Verification items for the finished model (mm, model axes). Face numbers are marked on the shaded views. A direction names the side the tool comes from. Coordinates: 2 decimals unless noted, no trailing zeros. Write each loop counter-clockwise with the first axis right and the second up, starting at its lowest first coordinate (ties: lowest second). Pieces come first, ordered by that corner, then holes. Notation, with made-up numbers: M 70,-34 L 93,-34 A12 ccw 93,-30 Z; hole C -34.75,66.25 d7. An arc over 180 degrees is marked long. Answer in a Markdown table with one row per item.
from build123d import *

# Parameters (mm, degrees)
F0_W     = 113
F0_H     = 67
F1_DEPTH = 2
F2_W     = 113
F2_H     = 67
F2_W_2   = 101
F2_H_2   = 55
F3_DEPTH = 10
F4_R     = 1.5
F5_DEPTH = 6.25


with BuildPart() as f1:
    # F0 (on Top) → F1 (new body)
    with BuildSketch(Plane.XY):
        Rectangle(F0_W, F0_H)
    extrude(amount=F1_DEPTH)

    # F2 (on face) → F3 (join)
    with BuildSketch(Plane.XY.offset(2)):
        Rectangle(F2_W, F2_H)
        Rectangle(F2_W_2, F2_H_2, mode=Mode.SUBTRACT)
    extrude(amount=F3_DEPTH)

    # F4 (on face) → F5 (cut)
    with BuildSketch(Plane.XY.offset(12)):
        with Locations((-36, 30.5)):
            Circle(F4_R)
        with Locations((-15, 30.5)):
            Circle(F4_R)
        with Locations((15, 30.5)):
            Circle(F4_R)
        with Locations((36, 30.5)):
            Circle(F4_R)
        with Locations((-15, -30.5)):
            Circle(F4_R)
        with Locations((-36, -30.5)):
            Circle(F4_R)
        with Locations((15, -30.5)):
            Circle(F4_R)
        with Locations((36, -30.5)):
            Circle(F4_R)
        with Locations((-53.5, 14)):
            Circle(F4_R)
        with Locations((-53.5, -14)):
            Circle(F4_R)
        with Locations((53.5, 14)):
            Circle(F4_R)
        with Locations((53.5, -14)):
            Circle(F4_R)
    extrude(amount=-F5_DEPTH, mode=Mode.SUBTRACT)


solid = f1.part
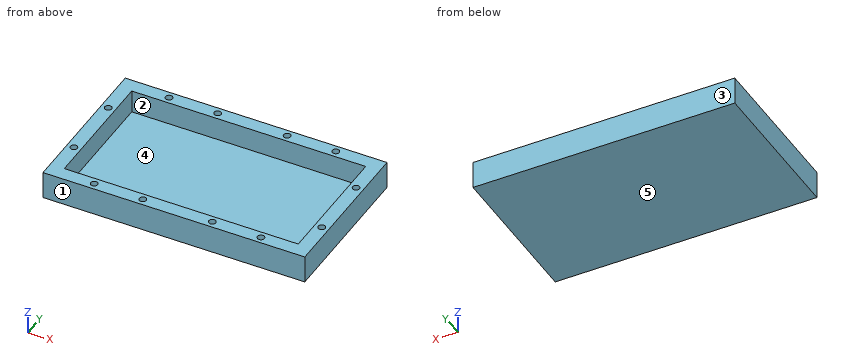
1) Sectioned sample at A-A (y = -14). Record the cut outline in (x, z), then the cut area to 4 significant figures.
Response values:
| item | result |
|---|---|
| outline | M -56.5,0 L 56.5,0 L 56.5,12 L 55,12 L 55,5.75 L 52,5.75 L 52,12 L 50.5,12 L 50.5,2 L -50.5,2 L -50.5,12 L -52,12 L -52,5.75 L -55,5.75 L -55,12 L -56.5,12 Z |
| area | 308.5 mm² |
2) Tool access check on the marked faces 1 and 2. Record the directions out of +Z, -Z, +X, -X, +Y, -Y that give a thin tool (end or side, any length) a straight path to the whole face; none if there is none.
Response values:
| item | result |
|---|---|
| face 1 | +Z, -Z, +X, -X, -Y |
| face 2 | +Z |
3) Sectioned sample at C-C (x = -53.5). Record the cut outline in (y, z), then the cut area to 4 significant figures.
Response values:
| item | result |
|---|---|
| outline | M -33.5,0 L 33.5,0 L 33.5,12 L 15.5,12 L 15.5,5.75 L 12.5,5.75 L 12.5,12 L -12.5,12 L -12.5,5.75 L -15.5,5.75 L -15.5,12 L -33.5,12 Z |
| area | 766.5 mm² |
4) Sectioned sample at B-B (z = 10). Give the number of separate pieces and of enclosed holes in the cut face, then the cut area to 3 significant figures.
Response values:
| item | result |
|---|---|
| separate pieces | 1 |
| enclosed holes | 13 |
| area | 1,930 mm² |
5) Release check for a two-part mould opening along Y. For the marked faces 3, 4 and 5 record: +Y half, -Y half, draft (parallel to the pull), parting line (faces both ways), or undercut.
Response values:
| item | result |
|---|---|
| face 3 | +Y half |
| face 4 | undercut |
| face 5 | draft |
6) Sectioned sample at D-D (z = 3.75). Record the cut outline in (x, y).
Response values:
| item | result |
|---|---|
| outline | M -56.5,-33.5 L 56.5,-33.5 L 56.5,33.5 L -56.5,33.5 Z; hole M -50.5,-27.5 L 50.5,-27.5 L 50.5,27.5 L -50.5,27.5 Z |
7) Thickness scan on L1, parallel to Y at x = 36, z = 9; L2, parallel to Y at x = -53.5, z = 7; L3, parallel to Y at x = 32, z = 6.25. Record the ranges inside material, lowest first. Write a range as [from, to].
Response values:
| item | result |
|---|---|
| L1 | y = [-33.5, -32], [-29, -27.5], [27.5, 29], [32, 33.5] |
| L2 | y = [-33.5, -15.5], [-12.5, 12.5], [15.5, 33.5] |
| L3 | y = [-33.5, -27.5], [27.5, 33.5] |
8) Depth check by flat-ended pin: pin 1 (4 mm diameter, centred on x = -33.5, y = 10, fed in from +Z); pin 2 (1.5 mm diameter, centred on x = -14.5, y = 30, fed in from +Z). Enter the tip coordinate at first touch or a pass-through.
Response values:
| item | result |
|---|---|
| pin 1 | stops at z = 2 |
| pin 2 | stops at z = 5.75 |
